Input: part model. Units: mm. Frame: model coordinates. Face numbers are marked on the shaded views. A direction names the side the tool comes from. Coordinates: 2 decimals unless noted, no trailing zeros.
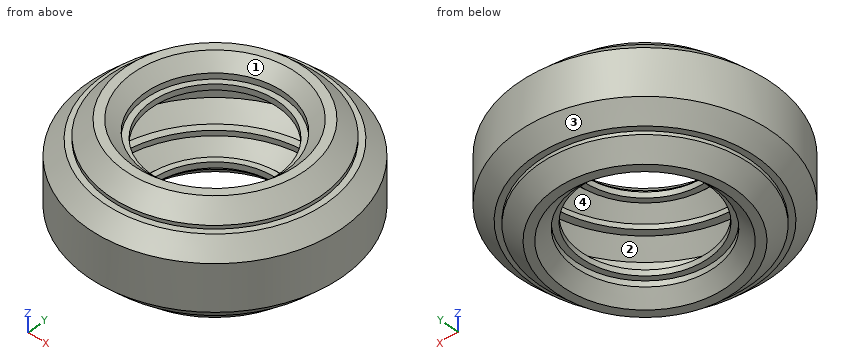
from build123d import *

# Parameters (mm, degrees)
EXTRUDE1_DEPTH      = 3.81
EXTRUDE2_DEPTH      = 0.508
CUT_EXTRUDE2_DEPTH  = 15.255714644
EXTRUDE3_DEPTH      = 3.302
EXTRUDE4_REACH      = 14.636
SKETCH9_W           = 3.553663376
SKETCH9_H           = 0.1905
SKETCH11_R          = 2.286
CUT_EXTRUDE3_DEPTH  = 13.636340451
SKETCH12_R          = 3.175
CUT_EXTRUDE4_DEPTH  = 0.508
SKETCH13_OUTSIDE_W  = 29.914
SKETCH13_OUTSIDE_H  = 14.674
SKETCH13_OUTSIDE_R  = 3.81
CUT_EXTRUDE5_DEPTH  = 15.255714644
CUT_EXTRUDE7_START  = 6.604
CUT_EXTRUDE7_DEPTH  = 6.604
SCALE1_SCALE_X      = 1
SCALE1_SCALE_Y      = 1
SCALE1_SCALE_Z      = 2.633333333
EXTRUDE6_DEPTH      = 30.24890252
EXTRUDE6_DEPTH_BACK = 30.24890252
SKETCH20_R          = 2.286
SKETCH21_R          = 12.7
SKETCH21_R_2        = 3.81
EXTRUDE7_DEPTH      = 10.16
EXTRUDE7_TAPER      = 35


# Read off the part's stored shape, not the designer's step: Shell1
with BuildPart() as part:
    # Sketch1 → Extrude1 (new body)
    with BuildSketch(Plane(origin=(0, 0, 0), x_dir=(1, 0, 0), z_dir=(0, 1, 0))):
        with BuildLine():
            Line((-7.62, 3.81), (0, 3.81))
            ThreePointArc((0, 3.81), (3.81, 0), (0, -3.81))
            Line((0, -3.81), (-7.62, -3.81))
            ThreePointArc((-7.62, -3.81), (-11.43, 0), (-7.62, 3.81))
        make_face()
    extrude(amount=EXTRUDE1_DEPTH)

    # Sketch4 → Extrude2 (add)
    with BuildSketch(Plane.XY.offset(3.81)):
        with BuildLine():
            Line((0, 0), (0, 3.81))
            Line((0, 3.81), (7.62, 3.81))
            ThreePointArc((7.62, 3.81), (10.314076836, 2.694076836), (11.43, 0))
            Line((11.43, 0), (7.62, 0))
            Line((7.62, 0), (0, 0))
        make_face()
    extrude2 = extrude(amount=-EXTRUDE2_DEPTH)

    # Sketch6 → Cut-Extrude2 (cut, through all)
    with BuildSketch(Plane.XY.offset(3.81)):
        with BuildLine():
            Line((6.858, 2.032), (6.858, 1.016))
            ThreePointArc((6.858, 1.016), (6.783605122, 0.836394878), (6.604, 0.762))
            Line((6.604, 0.762), (5.588, 0.762))
            ThreePointArc((5.588, 0.762), (5.408394878, 0.687605122), (5.334, 0.508))
            Line((5.334, 0.508), (5.334, -0.508))
            ThreePointArc((5.334, -0.508), (5.408394878, -0.687605122), (5.588, -0.762))
            Line((5.588, -0.762), (6.604, -0.762))
            ThreePointArc((6.604, -0.762), (6.783605122, -0.836394878), (6.858, -1.016))
            Line((6.858, -1.016), (6.858, -2.032))
            ThreePointArc((6.858, -2.032), (6.932394878, -2.211605122), (7.112, -2.286))
            Line((7.112, -2.286), (8.128, -2.286))
            ThreePointArc((8.128, -2.286), (8.307605122, -2.211605122), (8.382, -2.032))
            Line((8.382, -2.032), (8.382, -1.016))
            ThreePointArc((8.382, -1.016), (8.456394878, -0.836394878), (8.636, -0.762))
            Line((8.636, -0.762), (9.652, -0.762))
            ThreePointArc((9.652, -0.762), (9.831605122, -0.687605122), (9.906, -0.508))
            Line((9.906, -0.508), (9.906, 0.508))
            ThreePointArc((9.906, 0.508), (9.831605122, 0.687605122), (9.652, 0.762))
            Line((9.652, 0.762), (8.636, 0.762))
            ThreePointArc((8.636, 0.762), (8.456394878, 0.836394878), (8.382, 1.016))
            Line((8.382, 1.016), (8.382, 2.032))
            ThreePointArc((8.382, 2.032), (8.307605122, 2.211605122), (8.128, 2.286))
            Line((8.128, 2.286), (7.112, 2.286))
            ThreePointArc((7.112, 2.286), (6.932394878, 2.211605122), (6.858, 2.032))
        make_face()
    cut_extrude2 = extrude(amount=-CUT_EXTRUDE2_DEPTH, mode=Mode.SUBTRACT)

    # Sketch8 → Extrude3 (add)
    with BuildSketch(Plane(origin=(0, 0, 3.302), x_dir=(-1, 0, 0), z_dir=(0, 0, -1))):
        with BuildLine():
            Line((-10.795, 0), (-10.414, 0))
            ThreePointArc((-10.414, 0), (-9.726056742, 1.836017701), (-8.001, 2.767900829))
            Line((-8.001, 2.767900829), (-8.001, 3.152057106))
            ThreePointArc((-8.001, 3.152057106), (-9.995952441, 2.106056742), (-10.795, 0))
        make_face()
        with BuildLine():
            Line((-4.826, 0), (-4.445, 0))
            ThreePointArc((-4.445, 0), (-5.244047559, 2.106056742), (-7.239, 3.152057106))
            Line((-7.239, 3.152057106), (-7.239, 2.767900829))
            ThreePointArc((-7.239, 2.767900829), (-5.513943258, 1.836017701), (-4.826, 0))
        make_face()
    extrude3 = extrude(amount=EXTRUDE3_DEPTH)

    # Sketch9 → Extrude4 (add, up to next)
    with BuildSketch(Plane(origin=(0, 0, 0), x_dir=(-1, 0, 0), z_dir=(0, 0, -1)), mode=Mode.PRIVATE) as extrude4_sk1:
        with Locations((-2.858668312, 0.09525)):
            Rectangle(SKETCH9_W, SKETCH9_H)
    extrude4_tool1 = extrude(extrude4_sk1.sketch, amount=-EXTRUDE4_REACH, mode=Mode.PRIVATE) - part.part
    extrude4 = extrude4_tool1.solids().sort_by_distance((2.858668, 0.09525, 0))[0]
    add(extrude4)

    # Mirror5: Extrude2, Cut-Extrude2, Extrude3, Extrude4 across plane
    add(extrude2.mirror(Plane(origin=(7.62, 0, 0), x_dir=(1, 0, 0), z_dir=(0, 0, -1))))
    add(cut_extrude2.mirror(Plane(origin=(7.62, 0, 0), x_dir=(1, 0, 0), z_dir=(0, 0, -1))), mode=Mode.SUBTRACT)
    add(extrude3.mirror(Plane(origin=(7.62, 0, 0), x_dir=(1, 0, 0), z_dir=(0, 0, -1))))
    add(extrude4.mirror(Plane(origin=(7.62, 0, 0), x_dir=(1, 0, 0), z_dir=(0, 0, -1))))

    # Sketch11 → Cut-Extrude3 (cut, through all)
    with BuildSketch(Plane(origin=(0, 3.81, 0), x_dir=(1, 0, 0), z_dir=(0, 1, 0))):
        with Locations(Location((0, 0, 0), (0, 0, 270))):
            Circle(SKETCH11_R)
        with Locations(Location((-7.62, 0, 0), (0, 0, 270))):
            Circle(SKETCH11_R)
    extrude(amount=-CUT_EXTRUDE3_DEPTH, mode=Mode.SUBTRACT)

    # Sketch12 → Cut-Extrude4 (cut)
    with BuildSketch(Plane(origin=(0, 3.81, 0), x_dir=(1, 0, 0), z_dir=(0, 1, 0))):
        with Locations(Location((0, 0, 0), (0, 0, 270))):
            Circle(SKETCH12_R)
        with Locations(Location((-7.62, 0, 0), (0, 0, 270))):
            Circle(SKETCH12_R)
    extrude(amount=-CUT_EXTRUDE4_DEPTH, mode=Mode.SUBTRACT)

    # Mirror6: part across face


with BuildPart() as part_1:
    add(part.part)
    add(part.part.mirror(Plane(origin=(-2.524422527, 0, 0), x_dir=(0, 0, 1), z_dir=(0, -1, 0))))

    # Sketch13 outside → Cut-Extrude5 (cut, through all)
    with BuildSketch(Plane.XY.offset(3.81)):
        Rectangle(SKETCH13_OUTSIDE_W, SKETCH13_OUTSIDE_H)
        with Locations((7.62, 0)):
            Circle(SKETCH13_OUTSIDE_R, mode=Mode.SUBTRACT)
    extrude(amount=-CUT_EXTRUDE5_DEPTH, mode=Mode.SUBTRACT)

    # Sketch15 → Cut-Extrude7 (cut)
    with BuildSketch(Plane.XY.offset(-3.302).offset(CUT_EXTRUDE7_START)):
        with BuildLine():
            Line((4.486048338, 2.166667252), (5.299185915, 2.166667252))
            ThreePointArc((5.299185915, 2.166667252), (4.44500552, -0.00592023), (5.307282146, -2.175307134))
            Line((5.307282146, -2.175307134), (4.492039183, -2.175307134))
            ThreePointArc((4.492039183, -2.175307134), (3.810003627, -0.005256847), (4.486048338, 2.166667252))
        make_face()
    extrude(amount=-CUT_EXTRUDE7_DEPTH, mode=Mode.SUBTRACT)


with BuildPart() as part_2:
    # Scale1: scaled about (0, 0, 0)
    add(part_1.part.scale((SCALE1_SCALE_X, SCALE1_SCALE_Y, SCALE1_SCALE_Z), about=(0, 0, 0)))

    # Sketch17 → Revolve1 (revolve)
    with BuildSketch(Plane(origin=(0, 0, 0), x_dir=(1, 0, 0), z_dir=(0, 1, 0))):
        Polygon((10.414, 10.033), (10.414, -10.033), (22.86, -10.033), (22.86, -8.763), (21.59, -8.763), (21.59, -7.493), (22.86, -7.493), (22.86, -6.223), (21.59, -2.54), (21.59, 2.54), (22.86, 6.223), (22.86, 7.493), (21.59, 7.493), (21.59, 8.763), (22.86, 8.763), (22.86, 10.033), align=None)
    revolve(axis=Axis((7.62, 0, 0), (0, 0, -1)))

    # Sketch20 → Extrude6 (cut, two sides: drawn at the far end of the back side and taken through both)
    with BuildSketch(Plane.XY.offset(-EXTRUDE6_DEPTH_BACK)):
        with Locations((7.62, 7.62)):
            Circle(SKETCH20_R)
        with Locations((14.219113577, 3.81)):
            Circle(SKETCH20_R)
        with Locations((14.219113577, -3.81)):
            Circle(SKETCH20_R)
        with Locations((7.62, -7.62)):
            Circle(SKETCH20_R)
        with Locations((1.020886423, -3.81)):
            Circle(SKETCH20_R)
        with Locations((1.020886423, 3.81)):
            Circle(SKETCH20_R)
    extrude(amount=EXTRUDE6_DEPTH + EXTRUDE6_DEPTH_BACK, mode=Mode.SUBTRACT)

    # Sketch21 → Extrude7 (cut)
    with BuildSketch(Plane.XY.offset(10.033)):
        with Locations((7.62, 0)):
            Circle(SKETCH21_R)
        with Locations((7.62, 0)):
            Circle(SKETCH21_R_2, mode=Mode.SUBTRACT)
    extrude7 = extrude(amount=-EXTRUDE7_DEPTH, taper=EXTRUDE7_TAPER, mode=Mode.SUBTRACT)

    # Mirror7: Extrude7 across plane
    add(extrude7.mirror(Plane.XY), mode=Mode.SUBTRACT)


with BuildPart() as body_2:
    # Sketch22 → Revolve2 (revolve)
    with BuildSketch(Plane(origin=(0, 0, 0), x_dir=(1, 0, 0), z_dir=(0, 1, 0))):
        Polygon((22.86, -8.763), (22.86, -10.033), (25.527, -12.7), (27.432, -12.7), (30.861, -9.271), (30.861, -8.509), (32.131, -8.509), (35.56, -5.08), (35.56, 5.08), (32.131, 8.509), (30.861, 8.509), (30.861, 9.271), (27.432, 12.7), (25.527, 12.7), (22.86, 10.033), (22.86, 8.763), (21.59, 8.763), (21.59, 7.493), (22.86, 7.493), (22.86, 6.223), (21.59, 2.54), (21.59, -2.54), (22.86, -6.223), (22.86, -7.493), (21.59, -7.493), (21.59, -8.763), align=None)
    revolve(axis=Axis((7.62, 0, 0), (0, 0, -1)))

    # Shell1 outline → Shell1 (revolve, cut)
    with BuildSketch(Plane(origin=(7.62, 0, 0), x_dir=(1, 0, 0), z_dir=(0, -1, 0))):
        Polygon((15.24, -8.128), (15.875, -8.128), (15.875, -9.769974388), (18.170025612, -12.065), (19.548974388, -12.065), (22.606, -9.007974388), (22.606, -7.874), (24.247974388, -7.874), (27.305, -4.816974388), (27.305, 4.816974388), (24.247974388, 7.874), (22.606, 7.874), (22.606, 9.007974388), (19.548974388, 12.065), (18.170025612, 12.065), (15.875, 9.769974388), (15.875, 8.128), (15.24, 8.128), (15.24, 6.223), (13.97, 2.54), (13.97, -2.54), (15.24, -6.223), align=None)
    revolve(axis=Axis((7.62, 0, 0), (0, 0, 1)), mode=Mode.SUBTRACT)


solid = body_2.part
Item 1: Access query for the marked faces 1 and 2. Directions: +Z, -Z, +X, -X, +Y, -Y. A direction counts if a zero-diameter tool reaches every point of the face in a straight line with its end or side. Return the directions, or none.
Response values:
face 1: +Z
face 2: none
Item 2: Draft query along X for the marked faces 3 and 4. Return one class per face: pulls with the +X half, pulls with the -X half, needs draft (parallel to the pull), parting line crosses it, or undercut.
Response values:
face 3: parting line crosses it
face 4: undercut
Item 3: Ray query, probe 1 along Y at (x, z) = (7.62, -8.55) (3 decimals); probe 2 along Z at (x, y) = (-14, -7); probe 3 along Y at (x, z) = (-5.5, 9.25). Return the intervals inside material, ascending.
Response values:
probe 1: y = -23.241 to -22.606, -15.875 to -13.97, 13.97 to 15.875, 22.606 to 23.241
probe 2: z = -9.79 to -7.87, 7.87 to 9.79
probe 3: y = -19.18 to -18.11, -8.94 to -7.75, 7.75 to 8.94, 18.11 to 19.18
Item 4: Pin query (flat end, axial travel): pin 1 Ø24.5 at (x, y) = (4.5, -5) entering from +Z; pin 2 Ø3 at (y, z) = (19, 3) entering from +X; pin 3 Ø10 at (x, z) = (-7, 1.5) entering from +Y; pin 4 Ø10 at (x, z) = (26.5, 6.5) entering from +Y. Return the tip coordinate at first contact, or that it passes through.
Response values:
pin 1: stops at z = 12.7
pin 2: stops at x = 29.4
pin 3: stops at y = 26.23
pin 4: stops at y = 24.13
